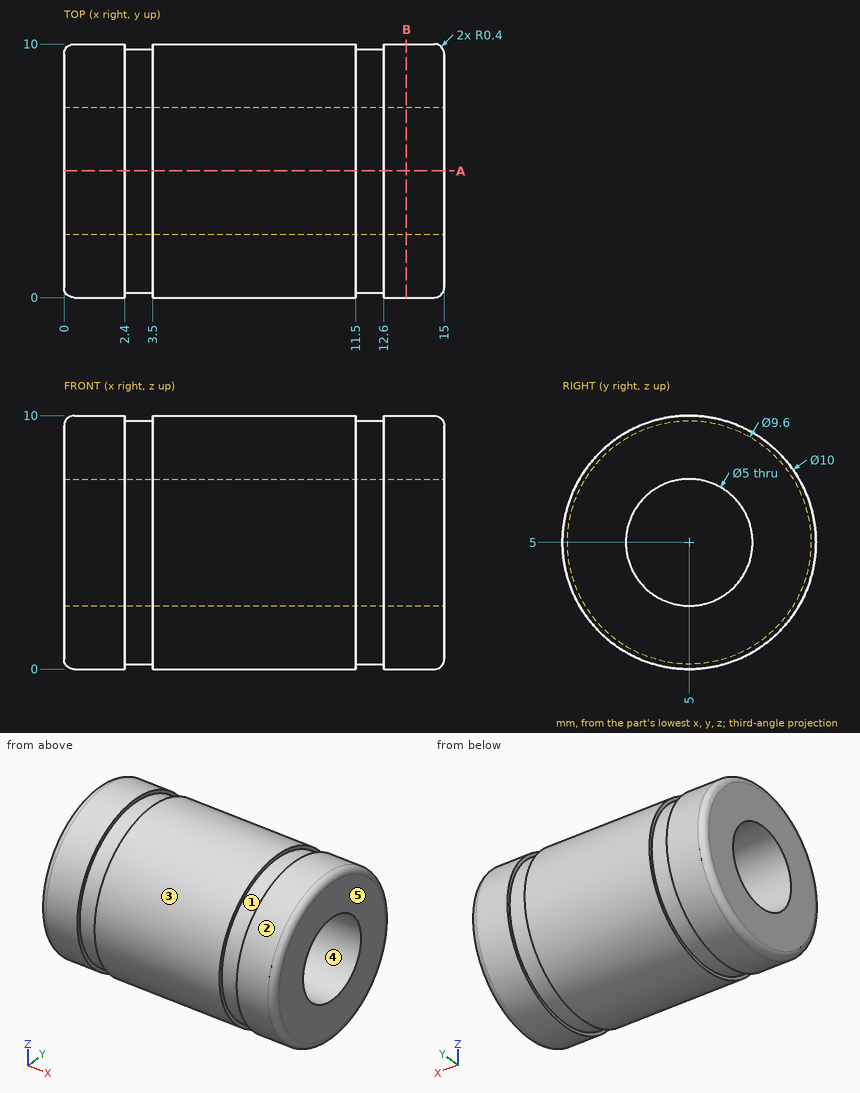
Input: dimensioned drawing with shaded views. Units: mm. Origin: part minimum x, y, z. A direction names the side the tool comes from. Coordinates: 2 decimals unless noted, no trailing zeros. Write each loop counter-clockwise with the first axis right and the second up, starting at its lowest first coordinate (ties: lowest second). Pieces come first, ordered by that corner, then holes. Notation, with made-up numbers: M 82,-26 L 89,-26 A15 cw 89,-18 Z; hole C 1,-24 d3. An arc over 180 degrees is marked long. Answer as a JSON object with one key per item and string values. Group by question number.
(1) Contact query for flat-ended pins moving along their axis: P1, Ø3, axis at x = 5.5, z = 8.5, coming from the -Y side; P2, Ø1.5, axis at x = 13, y = 7.5, coming from the -Z side; P3, Ø4, axis at x = 7.5, y = 1.5, coming from the +Z side. Output: stop coordinate, or through.
(2) Set-up query: the marked faces 1 and 2. Return all of +Z, -Z, +X, -X, +Y, -Y with unobstructed straight access to the full face (end or side cutting, diameter ignored); none if empty.
(3) Mould query, pull axis Z, two halves, no side actions, for the marked faces 3, 4 and 5. Classes: pulls with the +Z half, pulls with the -Z half, needs draft (parallel to the pull), parting line crosses it, or undercut.
(4) Ray query, line 1 along X through (y, z) = (0.5, 3.25); line 2 along Z through (x, y) = (6, 5); line 3 along Z through (x, y) = (12, 5). Return the intervals inside material, ascending. Write a range as [from, to].
(5) Section A-A on y = 5. Output: boundary loops of the cut face in (x, z), plus the area to 3 significant figures.
(6) Section B-B on x = 13.5. Output: boundary loops of the cut face in (y, z).
Result set:
{
 "1": {"P1": "stops at y = 0.42", "P2": "stops at z = 0.32", "P3": "stops at z = 9.77"},
 "2": {"face 1": "none", "face 2": "+X, -X"},
 "3": {"face 3": "parting line crosses it", "face 4": "undercut", "face 5": "needs draft"},
 "4": {"line 1": "x = [0.07, 2.4], [3.5, 11.5], [12.6, 14.93]", "line 2": "z = [0, 2.5], [7.5, 10]", "line 3": "z = [0.2, 2.5], [7.5, 9.8]"},
 "5": {"outline": "M 0,0.4 A0.4 ccw 0.4,0 L 2.4,0 L 2.4,0.2 L 3.5,0.2 L 3.5,0 L 11.5,0 L 11.5,0.2 L 12.6,0.2 L 12.6,0 L 14.6,0 A0.4 ccw 15,0.4 L 15,2.5 L 0,2.5 Z; M 0,7.5 L 15,7.5 L 15,9.6 A0.4 ccw 14.6,10 L 12.6,10 L 12.6,9.8 L 11.5,9.8 L 11.5,10 L 3.5,10 L 3.5,9.8 L 2.4,9.8 L 2.4,10 L 0.4,10 A0.4 ccw 0,9.6 Z", "area": "74.0 mm2"},
 "6": {"outline": "C 5,5 d10; hole C 5,5 d5"}
}
